The listing builds one solid part. Answer for the finished solid, in the listing's coordinates (mm). A direction names the side the tool comes from. Give positions to 0.01 mm unless a question says otherwise; leave off trailing zeros. Order: outer loops, then holes, each group sorted by start corner. A loop starts at its lowest first (then second) coordinate and runs counter-clockwise, first axis right, second up. Notation, with made-up numbers: (35, 9) -> (75, 9) arc R12 ccw to (75, 32) -> close; hole circle Ø2 at (51, 2). An arc over 180 degrees is marked (long way). One line per question, with ' | ' between items. Start each with the question number.
Autodesk Inventor part; units mm, degrees
ref_plane "YZ Plane" through (0, 0, 0) normal (1, 0, 0) x (0, 1, 0)
ref_plane "XZ Plane" through (0, 0, 0) normal (0, 1, 0) x (-1, 0, 0)
ref_plane "XY Plane" through (0, 0, 0) normal (0, 0, 1) x (1, 0, 0)
sketch "Skizze1" plane through (0, 0, 0) normal (0, 0, 1) x (1, 0, 0)
  line L0 (0, 15.4) -> (0, -15.4) construction
  line L1 (-15.4, 0) -> (15.4, 0) construction
  circle A0 centre (0, 0) radius 1.9
  arc A1 (-4.4, -4.1564) -> (4.4, -4.1564) centre (0, -2) ccw
  line L2 (0, 2) -> (0, 0) construction
  line L3 (0, 0) -> (2, 0) construction
  arc A2 (-4.4, -0.1564) -> (4.4, -0.1564) centre (0, 2) ccw
  arc A3 (4.4, 0.1564) -> (-4.4, 0.1564) centre (0, -2) ccw
  line L4 (0, 0) -> (0, -2) construction
  circle A4 centre (0, 0) radius 9.5
  circle A5 centre (0, 0) radius 11
  circle A6 centre (0, 0) radius 6.35 construction
  circle A7 centre (0, -6.35) radius 1.5
  circle A8 centre (0, 6.35) radius 1.5
  line L5 (0, -6.35) -> (0, 0) construction
  line L6 (0, 0) -> (-6.35, 0) construction
  line L7 (4.4, 4.1564) -> (4.4, -4.1564)
  line L8 (-4.4, 4.1564) -> (-4.4, -4.1564)
  line L9 (4.9, 2) -> (4.9, -2) construction
  arc A9 (4.4, 4.1564) -> (-4.4, 4.1564) centre (0, 2) ccw
  arc A10 (4.4, -0.1564) -> (4.4, 4.1564) centre (0, 2) ccw construction
  arc A11 (4.4, -4.1564) -> (4.4, 0.1564) centre (0, -2) ccw construction
  arc A12 (-4.4, 4.1564) -> (-4.4, -0.1564) centre (0, 2) ccw construction
  arc A13 (-4.4, 0.1564) -> (-4.4, -4.1564) centre (0, -2) ccw construction
  line L10 (-4.9, 2) -> (-4.9, -2) construction
  circle A14 centre (0, 0) radius 2.9
  circle A15 centre (0, 2) radius 5.9
  circle A16 centre (0, -6.35) radius 2.5
  circle A17 centre (0, 6.35) radius 2.5
  circle A18 centre (0, -2) radius 5.9
  circle A19 centre (0, 0) radius 4.9
  dimension "d0" = 3.8
  dimension "d1" = 2
  dimension "d14" = 2
  dimension "d15" = 180
  dimension "d16" = 9.5
  dimension "d17" = 1.5
  dimension "d20" = 6.35
  dimension "d21" = 3
  dimension "d26" = 0.5
  dimension "d27" = 0.5
  dimension "d28" = 4.9
  dimension "d31" = 1
  dimension "d34" = 1
  dimension "d37" = 1
  dimension "d40" = 1
extrude "Extrusion6" add sketch "Skizze1" along normal blind 3 contours A5
extrude "Extrusion7" add sketch "Skizze1" along normal blind 1.5 from surface at 3 contours A0 | L8 A19 A16 A1 | A1 A16 A18 A15 A19 L8 | A16 A19 A7 A1 | A1 A7 A16 A18 | A19 A15 L8 | L8 A15 A16 A19 | A7 A19 A1 | A1 A7 | A16 A15 A19 A7 | A18 A16 | A15 A19 A18 L8 | L8 A2 L7 A15 A16 | A15 A18 A19 | A7 A19 A16 A1 | A7 A19 | A16 A15 | A16 A1 L7 A19 A15 A18 | A15 A17 A9 L8 A19 A18 | L8 A3 A14 A2 | A19 L8 A18 | A16 A19 L7 A1 | A15 L7 A19 A16 | A17 A15 | A15 A17 A9 A8 | A14 A3 L7 A2 | A14 | L8 A18 A17 L7 A3 | L8 A19 A17 A18 | L8 A9 A17 A19 | A15 A19 L7 | L7 A18 A19 A15 | A18 A19 L7 A9 A17 A15 | A15 A19 A18 | A9 A8 A19 A17 | A18 A17 | A17 A19 A8 A18 | A18 L7 A19 | A9 A8 A19 | A8 A9 | A17 A19 L7 A18 | A19 A8 | A19 A17 A9 L7 | A17 A19 A8 A9 | A4 | A5
extrude "Extrusion15" add sketch "Skizze1" along normal blind 4 from surface at 4.5 contours A0 | A19 A15 L8 | L8 A15 A16 A19 | A16 A15 A19 A7 | A15 A19 A18 L8 | L8 A2 L7 A15 A16 | A7 A19 | A16 A15 | L8 A3 A14 A2 | A19 L8 A18 | A15 L7 A19 A16 | A14 A3 L7 A2 | A14 | L8 A18 A17 L7 A3 | L8 A19 A17 A18 | A15 A19 L7 | L7 A18 A19 A15 | A18 A17 | A17 A19 A8 A18 | A18 L7 A19 | A17 A19 L7 A18 | A19 A8
extrude "Extrusion8" cut sketch "Skizze1" along normal through all both and the other way through all contours A7 A19 A1 | A1 A7 | A7 A19 | A9 A8 A19 | A8 A9 | A19 A8
extrude "Extrusion16" add sketch "Skizze1" along normal blind 4 from surface at 8.5 contours A0 | L8 A3 A14 A2 | A14 A3 L7 A2 | A14
extrude "Extrusion12" cut sketch "Skizze1" along normal blind 3 from surface at 12.5 contours A16 A19 A7 A1 | A1 A7 A16 A18 | A16 A15 A19 A7 | A18 A16 | A7 A19 A16 A1 | A16 A15 | A17 A15 | A15 A17 A9 A8 | A9 A8 A19 A17 | A18 A17 | A17 A19 A8 A18 | A9 A8 A19 | A8 A9 | A19 A8 | A17 A19 A8 A9
extrude "Extrusion2" add sketch "Skizze1" along normal blind 4 from surface at 12.5 contours A0 | L8 A3 A14 A2 | A14 A3 L7 A2 | A14 | L8 A18 A17 L7 A3 | L8 A19 A17 A18 | L8 A9 A17 A19 | A9 A8 A19 A17 | A18 A17 | A17 A19 A8 A18 | A9 A8 A19 | A17 A19 L7 A18 | A19 A8 | A19 A17 A9 L7 | A17 A19 A8 A9
extrude "Extrusion3" add sketch "Skizze1" along normal blind 3 from surface at 16.5 contours A0 | L8 A3 A14 A2 | A14 A3 L7 A2 | A14
extrude "Extrusion4" add sketch "Skizze1" along normal blind 4 from surface at 19.5 contours A0 | L8 A19 A16 A1 | A16 A19 A7 A1 | L8 A15 A16 A19 | A7 A19 A1 | A16 A15 A19 A7 | L8 A2 L7 A15 A16 | A7 A19 A16 A1 | A7 A19 | A16 A15 | L8 A3 A14 A2 | A16 A19 L7 A1 | A15 L7 A19 A16 | A14 A3 L7 A2 | A14
extrude "Extrusion10" add sketch "Skizze1" along normal blind 5 from surface at 23.5 contours A0 | A14
extrude "Extrusion14" add sketch "Skizze1" along normal blind 4 from surface at 28.5 contours A0
equation "\"d14\" = d1"
equation "\"d27\" = d26"
properties part number "ExcentricShaft"
(1) Consider line 1 (Y direction, x = 0, z = 2.2); line 2 (Z direction, x = -4, y = 7.5); line 3 (Z direction, x = -0.25, y = 3.5). Determine where each line is inside the solid, lowest interval first.
(2) Given P1, Ø1, axis at x = 1, z = 23.5, coming from the +Y side; P2, Ø3, axis at y = -4.5, z = 26.5, coming from the +X side; P3, Ø4, axis at y = -1.5, z = 16, coming from the +X side; P4, Ø4, axis at x = 0, y = 6.35, coming from the -Z side, each flat-ended and moving along its own axis, determine where each tip first touches the part or whether it passes through.
(3) The part is cut by section C-C on y = -2.5. Determine the outline of the cut face in (x, z).
(4) The part is cut by section A-A on y = 5.5. Determine the outline of the cut face in (x, z), plus the area to 3 significant figures.
(5) For faces 4 (the face through (0, 4, 16.5)), 5 (the face through (-2.9, -0.1, 26)), 6 (the face through (0.1, -6.9, 21.5)), determine the directions among +Z, -Z, +X, -X, +Y, -Y from which every point of the face is accessible in a straight line to the end or side of a thin tool.
(6) The part is cut by section D-D on z = 25. Determine the outline of the cut face in (x, y).
(7) The part is cut by section B-B on x = -8.25. Determine the outline of the cut face in (y, z), plus the area to 3 significant figures.
(8) Determine the mould class of faces 1 (the face through (4.4, 0, 18)), 2 (the face through (-4.9, -0.1, 6.5)), 3 (the face through (4.38, 8.43, 1.48)) for opening direction X: pulls with the +X half, pulls with the -X half, needs draft (parallel to the pull), parting line crosses it, or undercut.
Result sheet:
1) line 1: y = -11 to -9.5, 9.5 to 11 | line 2: z = 3 to 4.5 | line 3: z = 3 to 8.5, 12.5 to 16.5
2) P1: stops at y = 2.87 | P2: passes through | P3: stops at x = 4.4 | P4: stops at z = 3
3) outline: (-10.71, 0) -> (-9.17, 0) -> (-9.17, 3) -> (9.17, 3) -> (9.17, 0) -> (10.71, 0) -> (10.71, 4.5) -> (4.21, 4.5) -> (4.21, 8.5) -> (1.94, 8.5) -> (1.94, 19.5) -> (4.4, 19.5) -> (4.4, 23.5) -> (1.47, 23.5) -> (1.47, 28.5) -> (-1.47, 28.5) -> (-1.47, 23.5) -> (-4.4, 23.5) -> (-4.4, 19.5) -> (-1.94, 19.5) -> (-1.94, 8.5) -> (-4.21, 8.5) -> (-4.21, 4.5) -> (-10.71, 4.5) -> close
4) outline: (-9.53, 0) -> (-7.75, 0) -> (-7.75, 3) -> (-1.24, 3) -> (-1.24, 4.5) -> (-9.53, 4.5) -> close; (-3.43, 12.5) -> (3.43, 12.5) -> (3.43, 16.5) -> (-3.43, 16.5) -> close; (1.24, 3) -> (7.75, 3) -> (7.75, 0) -> (9.53, 0) -> (9.53, 4.5) -> (1.24, 4.5) -> close | area: 63.0 mm^2
5) face 4: +Z, +Y | face 5: +Z | face 6: +Z, -Y
6) outline: circle Ø5.8 at (0, 0)
7) outline: (-7.28, 0) -> (-4.71, 0) -> (-4.71, 3) -> (4.71, 3) -> (4.71, 0) -> (7.28, 0) -> (7.28, 4.5) -> (-7.28, 4.5) -> close | area: 37.2 mm^2
8) face 1: pulls with the +X half | face 2: pulls with the -X half | face 3: undercut
